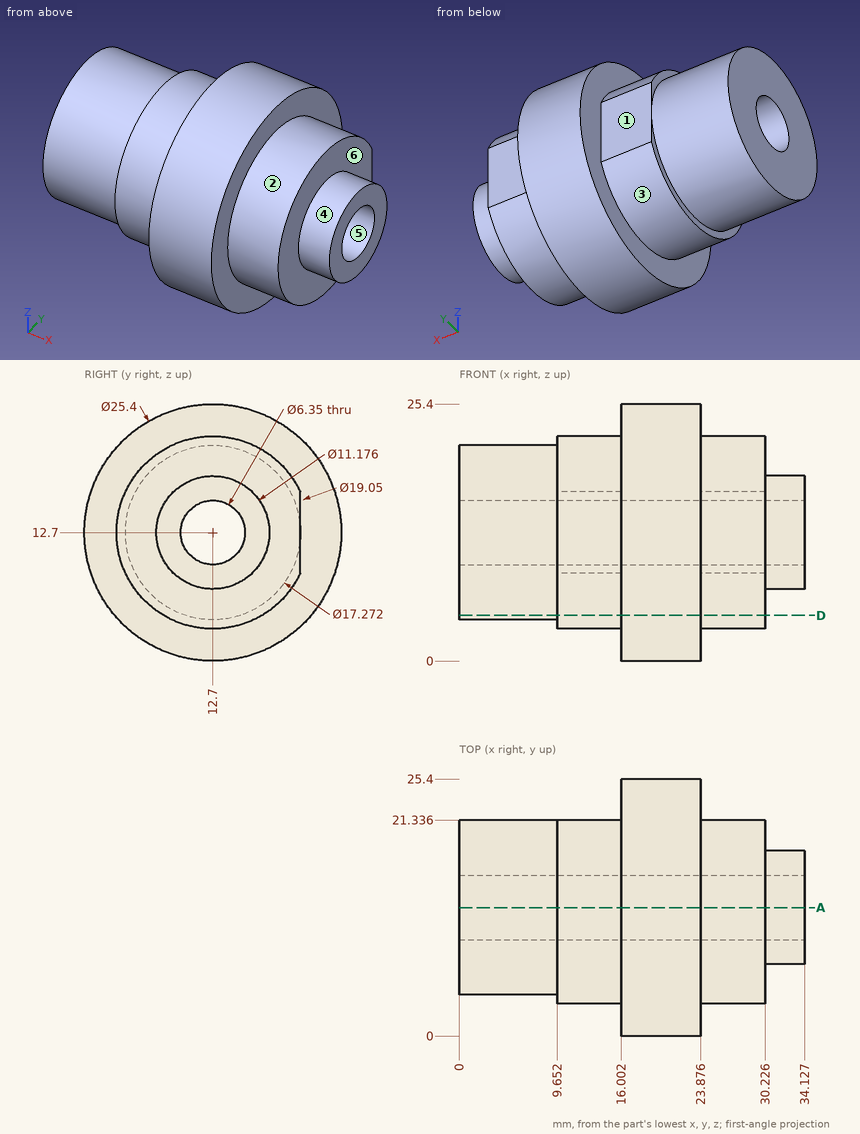
Can you work these out from the drawing? Everything is in mm from the part's minimum corner. A direction names the side the tool comes from. Round coordinates to 2 decimals unless told otherwise and drop trailing zeros. Loops run counter-clockwise (first coordinate to the right, second up) from the corner with the lowest first, then second, coordinate; pieces in that order, holes last.
1. For P1, Ø10, axis at x = 18.5, y = 4, coming from the +Z side; P2, Ø4, axis at x = 12, y = 6.5, coming from the -Z side; P3, Ø3, axis at x = 28.5, z = 12, coming from the +Y side, each with a flat end and sliding along its axis, tell me the tip position at first contact or that it passes through.
Answer list:
P1: stops at z = 24.85
P2: stops at z = 4.15
P3: stops at y = 21.34
2. We'd pull the mould along Z, two halves only. Please class the marked faces 4, 5 and 6: +Z half, -Z half, draft (parallel to the pull), parting line (faces both ways), or undercut.
Answer list:
face 4: parting line
face 5: undercut
face 6: draft
3. If we section it at A-A on y = 12.7: Write out the boundary of the cut face in (x, z) (1 decimal).
Answer list:
outline: (0, 4.1) - (9.7, 4.1) - (9.7, 3.2) - (16, 3.2) - (16, 0) - (23.9, 0) - (23.9, 3.2) - (30.2, 3.2) - (30.2, 7.1) - (34.1, 7.1) - (34.1, 9.5) - (0, 9.5) - close; (0, 15.9) - (34.1, 15.9) - (34.1, 18.3) - (30.2, 18.3) - (30.2, 22.2) - (23.9, 22.2) - (23.9, 25.4) - (16, 25.4) - (16, 22.2) - (9.7, 22.2) - (9.7, 21.3) - (0, 21.3) - close
4. If I drill on line 1 along Y through (x, z) = (18.5, 12.7) (1 decimal); line 2 along Z through (x, y) = (14, 12.7) (1 decimal); line 3 along Y through (x, z) = (26.5, 12.7) (1 decimal), over which ranges is the centre line in solid material (lowest first)?
Answer list:
line 1: y = 0 to 9.5, 15.9 to 25.4
line 2: z = 3.2 to 9.5, 15.9 to 22.2
line 3: y = 3.2 to 9.5, 15.9 to 21.3
5. If we section it at D-D on z = 4.5: Write out the boundary of the cut face in (x, y), plus the area to 3 significant figures.
Answer list:
outline: (0, 9.99) - (9.65, 9.99) - (9.65, 7.85) - (16, 7.85) - (16, 3) - (23.88, 3) - (23.88, 7.85) - (30.23, 7.85) - (30.23, 17.55) - (23.88, 17.55) - (23.88, 22.4) - (16, 22.4) - (16, 17.55) - (9.65, 17.55) - (9.65, 15.41) - (0, 15.41) - close
area: 328 mm2
6. Which directions (+Z, -Z, +X, -X, +Y, -Y) give clear straight access to the entire face, cutting with the end or side of a thin tool? Please do the marked faces 1, 2 and 3.
Answer list:
face 1: +Z, -Z, -X, +Y
face 2: +X
face 3: -X
